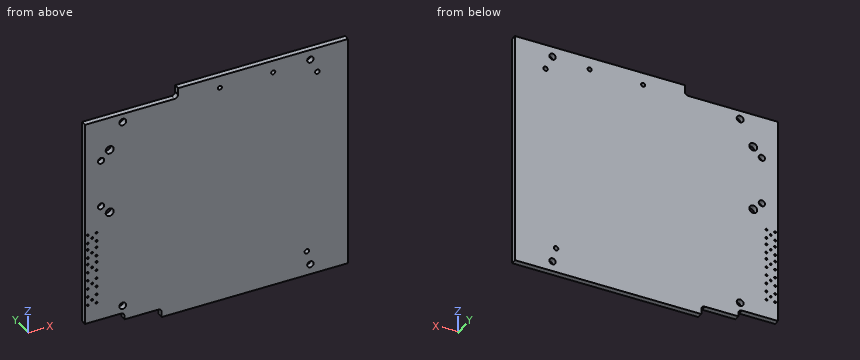
from build123d import *

# Parameters (mm, degrees)
SKETCH2_R           = 1
SKETCH2_R_2         = 1.15
SKETCH2_R_3         = 0.9
SKETCH2_R_4         = 0.595
SKETCH2_R_5         = 0.9271
SKETCH2_R_6         = 0.6604
SKETCH2_R_7         = 0.28
BOSS_EXTRUDE1_DEPTH = 1.6


with BuildPart() as part:
    # Sketch2 → Boss-Extrude1 (new body)
    with BuildSketch(Plane(origin=(0, 0, 0), x_dir=(1, 0, 0), z_dir=(0, 1, 0))):
        with BuildLine():
            Line((10.8682, -3), (10.9, -3))
            Line((10.9, -3), (10.9, -2.9682))
            Line((10.9, -2.9682), (10.9, 65.9682))
            Line((10.9, 65.9682), (10.9, 66))
            Line((10.9, 66), (10.8682, 66))
            Line((10.8682, 66), (-43.2683, 66))
            Line((-43.2683, 66), (-43.3, 66))
            Line((-43.3, 66), (-43.3, 65.9682))
            Line((-43.3, 65.9682), (-43.3, 64.431749961))
            ThreePointArc((-43.3, 64.431749961), (-43.277581689, 64.422432956), (-43.2683, 64.4))
            ThreePointArc((-43.2683, 64.4), (-43.277760728, 64.377389143), (-43.300504779, 64.368253257))
            ThreePointArc((-43.300504779, 64.368253257), (-43.5929, 63.6929), (-44.268253257, 63.400504779))
            ThreePointArc((-44.268253257, 63.400504779), (-44.277389143, 63.377760728), (-44.3, 63.3683))
            ThreePointArc((-44.3, 63.3683), (-44.322432956, 63.377581689), (-44.331749961, 63.4))
            Line((-44.331749961, 63.4), (-54.0682, 63.4))
            Line((-54.0682, 63.4), (-54.1, 63.4))
            Line((-54.1, 63.4), (-54.1, 63.3683))
            Line((-54.1, 63.3683), (-54.1, 62.3318))
            ThreePointArc((-54.1, 62.3318), (-54.077514004, 62.322485996), (-54.0682, 62.3))
            ThreePointArc((-54.0682, 62.3), (-54.077693743, 62.277335692), (-54.100506344, 62.268204031))
            ThreePointArc((-54.100506344, 62.268204031), (-54.392917413, 61.592882587), (-55.068253257, 61.300504779))
            ThreePointArc((-55.068253257, 61.300504779), (-55.077389143, 61.277760728), (-55.1, 61.2683))
            ThreePointArc((-55.1, 61.2683), (-55.122432956, 61.277581689), (-55.131749961, 61.3))
            Line((-55.131749961, 61.3), (-65.5683, 61.3))
            Line((-65.5683, 61.3), (-65.6, 61.3))
            Line((-65.6, 61.3), (-65.6, 61.2683))
            Line((-65.6, 61.2683), (-65.6, 0.0318))
            Line((-65.6, 0.0318), (-65.6, 0))
            Line((-65.6, 0), (-65.5683, 0))
            Line((-65.5683, 0), (-39.5318, 0))
            ThreePointArc((-39.5318, 0), (-39.522485996, 0.022485996), (-39.5, 0.0318))
            ThreePointArc((-39.5, 0.0318), (-39.477335692, 0.022306257), (-39.468204031, -0.000506344))
            ThreePointArc((-39.468204031, -0.000506344), (-38.7929, -0.2929), (-38.500506344, -0.968204031))
            ThreePointArc((-38.500506344, -0.968204031), (-38.477693743, -0.977335692), (-38.4682, -1))
            ThreePointArc((-38.4682, -1), (-38.477514004, -1.022485996), (-38.5, -1.0318))
            Line((-38.5, -1.0318), (-38.5, -2.9682))
            Line((-38.5, -2.9682), (-38.5, -3))
            Line((-38.5, -3), (-38.4682, -3))
            Line((-38.4682, -3), (10.8682, -3))
        make_face()
        with Locations(Location((-54.6, 2.5, 0), (0, 0, 270))):
            Circle(SKETCH2_R, mode=Mode.SUBTRACT)
        with Locations(Location((-58.4, 9.9, 0), (0, 0, 270))):
            Circle(SKETCH2_R_2, mode=Mode.SUBTRACT)
        with Locations(Location((-60.9, 12.5, 0), (0, 0, 270))):
            Circle(SKETCH2_R_3, mode=Mode.SUBTRACT)
        with Locations(Location((-60.9, 26.5, 0), (0, 0, 270))):
            Circle(SKETCH2_R_3, mode=Mode.SUBTRACT)
        with Locations(Location((-58.4, 29.1, 0), (0, 0, 270))):
            Circle(SKETCH2_R_2, mode=Mode.SUBTRACT)
        with Locations(Location((-26.37, 0.6, 0), (0, 0, 270))):
            Circle(SKETCH2_R_4, mode=Mode.SUBTRACT)
        with Locations(Location((-10.83, 0.6, 0), (0, 0, 270))):
            Circle(SKETCH2_R_4, mode=Mode.SUBTRACT)
        with Locations(Location((-0.032, 0.004, 0), (0, 0, 270))):
            Circle(SKETCH2_R_5, mode=Mode.SUBTRACT)
        with Locations(Location((2, 4.3347, 0), (0, 0, 270))):
            Circle(SKETCH2_R_6, mode=Mode.SUBTRACT)
        with Locations(Location((-64.77, 34.23, 0), (0, 0, 270))):
            Circle(SKETCH2_R_7, mode=Mode.SUBTRACT)
        with Locations(Location((-63.5, 35.5, 0), (0, 0, 270))):
            Circle(SKETCH2_R_7, mode=Mode.SUBTRACT)
        with Locations(Location((-62.23, 34.23, 0), (0, 0, 270))):
            Circle(SKETCH2_R_7, mode=Mode.SUBTRACT)
        with Locations(Location((-64.77, 36.77, 0), (0, 0, 270))):
            Circle(SKETCH2_R_7, mode=Mode.SUBTRACT)
        with Locations(Location((-62.23, 36.77, 0), (0, 0, 270))):
            Circle(SKETCH2_R_7, mode=Mode.SUBTRACT)
        with Locations(Location((-64.77, 38.73, 0), (0, 0, 270))):
            Circle(SKETCH2_R_7, mode=Mode.SUBTRACT)
        with Locations(Location((-63.5, 40, 0), (0, 0, 270))):
            Circle(SKETCH2_R_7, mode=Mode.SUBTRACT)
        with Locations(Location((-62.23, 38.73, 0), (0, 0, 270))):
            Circle(SKETCH2_R_7, mode=Mode.SUBTRACT)
        with Locations(Location((-64.77, 41.27, 0), (0, 0, 270))):
            Circle(SKETCH2_R_7, mode=Mode.SUBTRACT)
        with Locations(Location((-62.23, 41.27, 0), (0, 0, 270))):
            Circle(SKETCH2_R_7, mode=Mode.SUBTRACT)
        with Locations(Location((-64.77, 43.23, 0), (0, 0, 270))):
            Circle(SKETCH2_R_7, mode=Mode.SUBTRACT)
        with Locations(Location((-62.23, 43.23, 0), (0, 0, 270))):
            Circle(SKETCH2_R_7, mode=Mode.SUBTRACT)
        with Locations(Location((-63.5, 44.5, 0), (0, 0, 270))):
            Circle(SKETCH2_R_7, mode=Mode.SUBTRACT)
        with Locations(Location((-64.77, 45.77, 0), (0, 0, 270))):
            Circle(SKETCH2_R_7, mode=Mode.SUBTRACT)
        with Locations(Location((-62.23, 45.77, 0), (0, 0, 270))):
            Circle(SKETCH2_R_7, mode=Mode.SUBTRACT)
        with Locations(Location((-64.77, 48.23, 0), (0, 0, 270))):
            Circle(SKETCH2_R_7, mode=Mode.SUBTRACT)
        with Locations(Location((-62.23, 48.23, 0), (0, 0, 270))):
            Circle(SKETCH2_R_7, mode=Mode.SUBTRACT)
        with Locations(Location((-63.5, 49.5, 0), (0, 0, 270))):
            Circle(SKETCH2_R_7, mode=Mode.SUBTRACT)
        with Locations(Location((-64.77, 50.77, 0), (0, 0, 270))):
            Circle(SKETCH2_R_7, mode=Mode.SUBTRACT)
        with Locations(Location((-62.23, 50.77, 0), (0, 0, 270))):
            Circle(SKETCH2_R_7, mode=Mode.SUBTRACT)
        with Locations(Location((-64.77, 53.23, 0), (0, 0, 270))):
            Circle(SKETCH2_R_7, mode=Mode.SUBTRACT)
        with Locations(Location((-63.5, 54.5, 0), (0, 0, 270))):
            Circle(SKETCH2_R_7, mode=Mode.SUBTRACT)
        with Locations(Location((-62.23, 53.23, 0), (0, 0, 270))):
            Circle(SKETCH2_R_7, mode=Mode.SUBTRACT)
        with Locations(Location((-64.77, 55.77, 0), (0, 0, 270))):
            Circle(SKETCH2_R_7, mode=Mode.SUBTRACT)
        with Locations(Location((-62.23, 55.77, 0), (0, 0, 270))):
            Circle(SKETCH2_R_7, mode=Mode.SUBTRACT)
        with Locations(Location((-54.6, 59.05, 0), (0, 0, 270))):
            Circle(SKETCH2_R, mode=Mode.SUBTRACT)
        with Locations(Location((-1.05, 58.6907, 0), (0, 0, 270))):
            Circle(SKETCH2_R_6, mode=Mode.SUBTRACT)
        with Locations(Location((-0.032, 62.996, 0), (0, 0, 270))):
            Circle(SKETCH2_R_5, mode=Mode.SUBTRACT)
    extrude(amount=BOSS_EXTRUDE1_DEPTH)


solid = part.part
CAD build for the part. Positions are in the model's coordinates, mm. Coordinates: 2 decimals unless noted, no trailing zeros. Order: outer loops, then holes, each group sorted by start corner. A loop starts at its lowest first (then second) coordinate and runs counter-clockwise, first axis right, second up. Notation, with made-up numbers: (9.5, 1.5) -> (58.5, 1.5) arc R23 ccw to (58.5, 33.5) -> close; hole circle Ø3 at (34, 8.25). An arc over 180 degrees is marked (long way). Answer in a Markdown table with one row per item.
1) Band-saw the part on A-A (x = -52). List the corners of the cut face in (y, z), and give its area (3 significant figures).
Check values:
| item | result |
|---|---|
| outline | (0, -63.4) -> (1.6, -63.4) -> (1.6, 0) -> (0, 0) -> close |
| area | 101 mm2 |
2) Drill centre lines: line 1 (X direction, y = 1, z = -41.27); line 2 (X direction, y = 1.2, z = -29.1); line 3 (X direction, y = 1.05, z = -35.5). Where is each one in solid material? Low to high.
Check values:
| item | result |
|---|---|
| line 1 | -65.6 to -65.05, -64.49 to -62.51, -61.95 to 10.9 |
| line 2 | -65.6 to -59.55, -57.25 to 10.9 |
| line 3 | -65.6 to -63.78, -63.22 to 10.9 |
3) Flat gauge pins, fed straight in: P1, Ø0.8, axis at y = 0.5, z = -65, coming from the -X side; P2, Ø0.8, axis at x = -60, y = 1, coming from the -Z side; P3, Ø0.5, axis at x = -52.5, y = 1, coming from the +Z side. Where does each tip first touch, or does it go through?
Check values:
| item | result |
|---|---|
| P1 | x = -43.3 |
| P2 | z = -61.3 |
| P3 | z = 0 |
4) Band-saw the part on B-B (y = 1.3). Give the number of separate pieces and of enclosed holes in the cut face, and give its area (3 significant figures).
Check values:
| item | result |
|---|---|
| separate pieces | 1 |
| enclosed holes | 37 |
| area | 5,080 mm2 |
